Source: CAD feature listing. Evaluate the final solid. Frame: model axes, mm. A direction names the side the tool comes from. Coordinates: 2 decimals unless noted, no trailing zeros. Order: outer loops, then holes, each group sorted by start corner. A loop starts at its lowest first (then second) coordinate and runs counter-clockwise, first axis right, second up.
```python
from build123d import *

# Parameters (mm, degrees)
F0_W     = 4.5
F0_H     = 3
F0_R     = 0.75
F1_DEPTH = 10
F2_R     = 1
F3_DEPTH = 4
F4_R     = 1
F5_DEPTH = 4
F6_W     = 4
F6_H     = 10
F6_R     = 1
F7_DEPTH = 2
F8_W     = 4
F8_H     = 10
F8_R     = 1
F9_DEPTH = 2
F10_R    = 0.99999


# Not quite as in the source:
# - a fillet or chamfer is up to 0.001 mm smaller than in the source, because OpenCascade refuses the exact size


with BuildPart() as f1:
    # F0 (on Front) → F1 (new body)
    with BuildSketch(Plane.XZ):
        Polygon((-13, 4), (-13, 0), (-7, 0), (-7, 2), (7, 2), (7, 0), (13, 0), (13, 4), (2.25, 4), (-2.25, 4), align=None)
        with Locations((0, 5.5)):
            Rectangle(F0_W, F0_H)
        with Locations((0, 5)):
            Circle(F0_R, mode=Mode.SUBTRACT)
    extrude(amount=F1_DEPTH)

    # F2 (on face) → F3 (cut)
    with BuildSketch(Plane.XY.offset(4)):
        with Locations((-11, -2)):
            Circle(F2_R)
        with Locations((-11, -8)):
            Circle(F2_R)
    extrude(amount=-F3_DEPTH, mode=Mode.SUBTRACT)

    # F4 (on face) → F5 (cut)
    with BuildSketch(Plane.XY.offset(4)):
        with Locations((11, -2)):
            Circle(F4_R)
        with Locations((11, -8)):
            Circle(F4_R)
    extrude(amount=-F5_DEPTH, mode=Mode.SUBTRACT)

    # F6 (on face) → F7 (cut)
    with BuildSketch(Plane.XY.offset(4)):
        with Locations((-11, -5)):
            Rectangle(F6_W, F6_H)
        with Locations((-11, -8)):
            Circle(F6_R, mode=Mode.SUBTRACT)
        with Locations((-11, -2)):
            Circle(F6_R, mode=Mode.SUBTRACT)
    extrude(amount=-F7_DEPTH, mode=Mode.SUBTRACT)

    # F8 (on face) → F9 (cut)
    with BuildSketch(Plane.XY.offset(4)):
        with Locations((11, -5)):
            Rectangle(F8_W, F8_H)
        with Locations((11, -8)):
            Circle(F8_R, mode=Mode.SUBTRACT)
        with Locations((11, -2)):
            Circle(F8_R, mode=Mode.SUBTRACT)
    extrude(amount=-F9_DEPTH, mode=Mode.SUBTRACT)

    # F10 (radius 1 in the source; OpenCascade refuses exactly that, so slightly less here)
    f10_edges = [f1.edges().sort_by_distance(p)[0] for p in [
        (-9, -5, 4),
        (-2.25, -5, 7),
        (-2.25, -5, 4),
        (2.25, -5, 7),
        (2.25, -5, 4),
        (9, -5, 4),
        (-13, -5, 2),
        (13, -5, 2),
    ]]
    fillet(f10_edges, radius=F10_R)


solid = f1.part
```
Q1. Set-up query: faces 4 (the flat face through (10, -5, 0)), 5 (the flat face through (-9, -5.1, 2.5)), 6 (the flat face through (9, -5.1, 2.5)). Return all of +Z, -Z, +X, -X, +Y, -Y with unobstructed straight access to the full face (end or side cutting, diameter ignored); none if empty.
Solutions:
face 4: -Z, +X, -X, +Y, -Y
face 5: +Z, -X, +Y, -Y
face 6: +Z, +X, +Y, -Y
Q2. Pin query (flat end, axial travel): P1, Ø3.5, axis at x = -10, y = -6.5, coming from the +Z side; P2, Ø1.8, axis at x = 11, y = -2, coming from the +Z side; P3, Ø4, axis at x = 4.5, y = -7, coming from the +Z side; P4, Ø3.5, axis at x = 10.5, y = -3.5, coming from the +Z side. Return the tip coordinate at first contact, or that it passes through.
Solutions:
P1: stops at z = 3.97
P2: passes through
P3: stops at z = 4.34
P4: stops at z = 3.66
Q3. Section query C-C on x = -11. Output: boundary loops of the cut face in (y, z).
Solutions:
outline: (-10, 0) - (-9, 0) - (-9, 2) - (-10, 2) - close; (-7, 0) - (-3, 0) - (-3, 2) - (-7, 2) - close; (-1, 0) - (0, 0) - (0, 2) - (-1, 2) - close
Q4. Material intervals for line 1 along Y through (x, z) = (11, 1); line 2 along Z through (x, y) = (0, -5.25); line 3 along X through (y, z) = (-4, 1), sorted ascending.
Solutions:
line 1: y = -10 to -9, -7 to -3, -1 to 0
line 2: z = 2 to 4.25, 5.75 to 7
line 3: x = -13 to -7, 7 to 13
Q5. Section query D-D on y = -0.25. Output: boundary loops of the cut face in (x, z).
Solutions:
outline: (-13, 0) - (-7, 0) - (-7, 2) - (7, 2) - (7, 0) - (13, 0) - (13, 1) arc R1 ccw to (12, 2) - (9, 2) - (9, 3) arc R1 ccw to (8, 4) - (3.25, 4) arc R1 cw to (2.25, 5) - (2.25, 6) arc R1 ccw to (1.25, 7) - (-1.25, 7) arc R1 ccw to (-2.25, 6) - (-2.25, 5) arc R1 cw to (-3.25, 4) - (-8, 4) arc R1 ccw to (-9, 3) - (-9, 2) - (-12, 2) arc R1 ccw to (-13, 1) - close; hole circle Ø1.5 at (0, 5)
Q6. Pull-direction query (Y, two-part tool) for faces 1 (the flat face through (-2.25, -4.9, 5.5)), 2 (the cylindrical face through (-11, -7, 1)), 3 (the flat face through (-0.1, 0, 2.5)); classes: pulls with the +Y half, pulls with the -Y half, needs draft (parallel to the pull), parting line crosses it, or undercut.
Solutions:
face 1: needs draft
face 2: undercut
face 3: pulls with the +Y half
Q7. Section query B-B on y = -2. Give the number of separate pieces and of enclosed holes in the cut face, plus the area to 3 significant figures.
Solutions:
separate pieces: 3
enclosed holes: 1
area: 62.9 mm2
Q8. Section query A-A on z = 0.75. Output: boundary loops of the cut face in (x, y).
Solutions:
outline: (-13, -10) - (-7, -10) - (-7, 0) - (-13, 0) - close; (7, -10) - (13, -10) - (13, 0) - (7, 0) - close; hole circle Ø2 at (-11, -8); hole circle Ø2 at (-11, -2); hole circle Ø2 at (11, -8); hole circle Ø2 at (11, -2)
